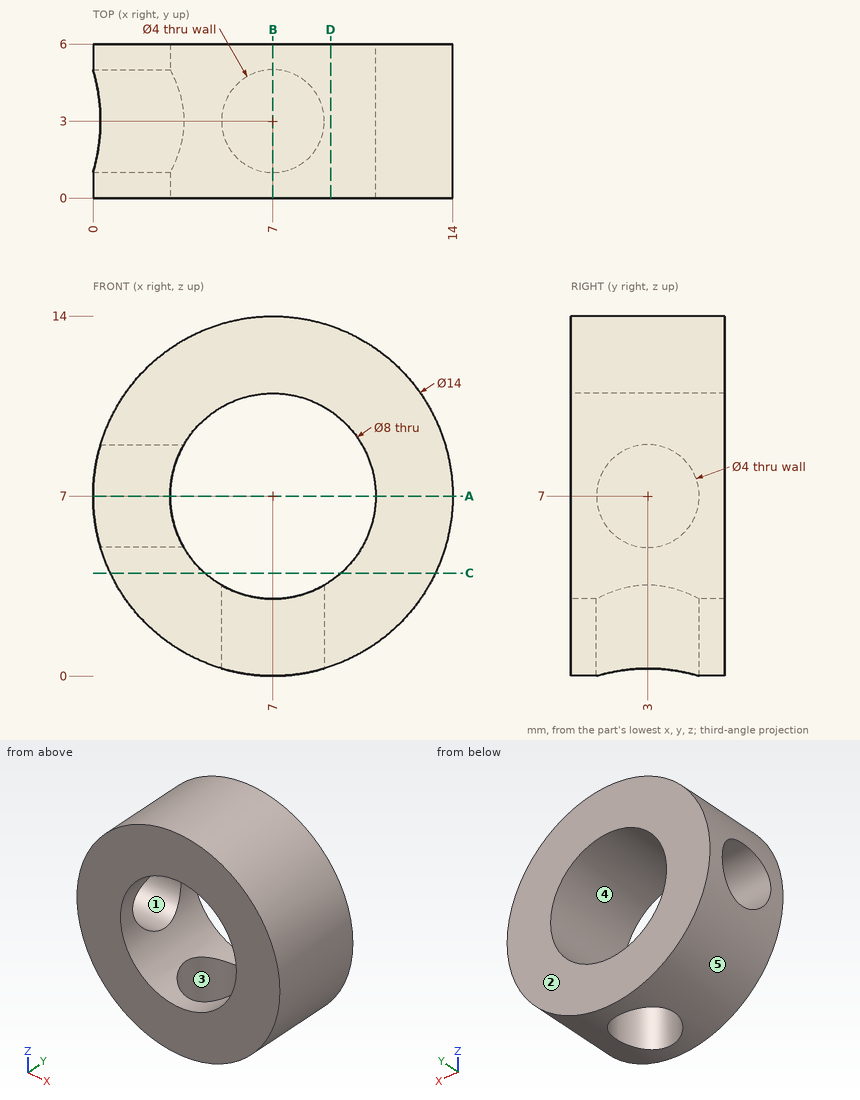
Print and shaded views of the part. All mm, measured from the part's lowest x, y and z. A direction names the side the tool comes from. Coordinates: 2 decimals unless noted, no trailing zeros. Write each loop counter-clockwise with the first axis right and the second up, starting at its lowest first coordinate (ties: lowest second). Pieces come first, ordered by that corner, then holes.
(1) Drill centre lines: probe 1 along Y at (x, z) = (7, 1.15); probe 2 along Z at (x, y) = (7, 3); probe 3 along Z at (x, y) = (4, 2.75). Where is each one in solid material? Low to high.
(2) Cut at C-C, the plane z = 4. List the corners of the cut face in (x, y).
(3) Flat gauge pins, fed straight in: pin 1 (3 mm diameter, centred on x = 3, y = 1.5, fed in from -Z); pin 2 (1 mm diameter, centred on x = 2.5, y = 5.5, fed in from -Z); pin 3 (3.5 mm diameter, centred on y = 3, z = 7, fed in from -X). Where does each tip first touch, or does it go through?
(4) 3-axis set-ups, long thin cutter, end or side, ignore diameter. For the marked faces 1 and 2: which of +Z, -Z, +X, -X, +Y, -Y reach the whole face in a straight line?
(5) Cut at D-D, the plane x = 9.25. List the corners of the cut face in (y, z), and give its area (3 significant figures).
(6) Cut at B-B, the plane x = 7. List the corners of the cut face in (y, z), and give its area (3 significant figures).
(7) Two-plate mould, pull along Z, no slides. Class the marked faces 3, 4 and 5: +Z half, -Z half, draft (parallel to the pull), parting line (faces both ways), or undercut.
(8) Cut at A-A, the plane z = 7. List the corners of the cut face in (x, y).
Geometry says:
1. probe 1: y = 0 to 1, 5 to 6
1. probe 2: z = 11 to 14
1. probe 3: z = 0.68 to 4.35, 9.65 to 13.32
2. outline: (0.68, 0) - (4.35, 0) - (4.35, 6) - (0.68, 6) - close; (9.65, 0) - (13.32, 0) - (13.32, 6) - (9.65, 6) - close
3. pin 1: stops at z = 0.46
3. pin 2: stops at z = 1.26
3. pin 3: stops at x = 10.6
4. face 1: -X
4. face 2: +Z, -Z, +X, -X, +Y
5. outline: (0, 0.37) - (6, 0.37) - (6, 3.69) - (0, 3.69) - close; (0, 10.31) - (6, 10.31) - (6, 13.63) - (0, 13.63) - close
5. area: 39.9 mm2
6. outline: (0, 0) - (1, 0) - (1, 3) - (0, 3) - close; (0, 11) - (6, 11) - (6, 14) - (0, 14) - close; (5, 0) - (6, 0) - (6, 3) - (5, 3) - close
6. area: 24.0 mm2
7. face 3: draft
7. face 4: undercut
7. face 5: parting line
8. outline: (0, 0) - (3, 0) - (3, 1) - (0, 1) - close; (0, 5) - (3, 5) - (3, 6) - (0, 6) - close; (11, 0) - (14, 0) - (14, 6) - (11, 6) - close
